The listing builds one solid part. Answer for the finished solid, in the listing's coordinates (mm). Face numbers are marked on the shaded views. Round coordinates to 2 decimals unless told otherwise and drop trailing zeros. Write each loop counter-clockwise with the first axis right and the second up, starting at its lowest first coordinate (ties: lowest second). Pieces come first, ordered by that corner, then holes. Notation, with made-up numbers: M 85.5,-39 L 105.5,-39 A20 ccw 105.5,-33 Z; hole C 16,78.5 d10. An arc over 180 degrees is marked long. One line per item, written item: value. Start each with the question number.
(1) Given P1, Ø8, axis at x = -11.5, z = 9, coming from the -Y side; P2, Ø9.5, axis at x = 22.5, z = 10.5, coming from the -Y side, each flat-ended and moving along its own axis, determine where each tip first touches the part or whether it passes through.
(2) Section A-A (y = -97.5) is taken. Determine the outline of the cut face in (x, z).
(3) Section D-D (z = 29.5) is taken. Determine the outline of the cut face in (x, y).
(4) For a pull along Z with two mould halves and no side action, classify the marked faces 1, 2, 3 and 4 as released by +Z, released by -Z, zero draft, split by the parting line, or undercut.
(5) Section B-B (x = 12) is taken. Determine the outline of the cut face in (y, z).
(6) Consider probe 1 along Y at (x, z) = (-2.5, 4); probe 2 along Y at (x, z) = (12.5, 7); probe 3 along Z at (x, y) = (78.5, -28). Determine where each line is inside the solid, lowest interval first.
(7) Section C-C (y = -52.5) is taken. Determine the outline of the cut face in (x, z), plus the area to 3 significant figures.
```python
from build123d import *

# Parameters (mm, degrees)
F0_W     = 150
F0_H     = 100
F1_DEPTH = 100
F4_DEPTH = 25
F5_SIZE  = 24
F6_R     = 9.380877
F7_DEPTH = 24.5
F8_W     = 13.083855
F8_H     = 15.305644
F9_DEPTH = 25.7


with BuildPart() as f1:
    # F0 (on Front) → F1 (new body)
    with BuildSketch(Plane.XZ):
        with Locations((15.379184, 8.105334)):
            Rectangle(F0_W, F0_H)
    extrude(amount=F1_DEPTH)

    # F3 (on face) → F4 (join)
    with BuildSketch(Plane.XZ.offset(100)):
        with BuildLine():
            ThreePointArc((-14.94097, 58.105334), (10.023203, 33.033909), (35.058928, 58.033884))
            ThreePointArc((35.058928, 58.033884), (35.058903, 58.069609), (35.058826, 58.105334))
            Line((35.058826, 58.105334), (-14.94097, 58.105334))
        make_face()
    extrude(amount=F4_DEPTH)

    # F5
    f5_edges = [f1.edges().sort_by_distance(p)[0] for p in [
        (90.379184, -50, 58.105334),
    ]]
    chamfer(f5_edges, length=F5_SIZE)

    # F6 (on face) → F7 (cut)
    with BuildSketch(Plane.XZ.offset(100)):
        with Locations((19.53912, 7.652821)):
            Circle(F6_R)
    extrude(amount=-F7_DEPTH, mode=Mode.SUBTRACT)

    # F8 (on face) → F9 (cut)
    with BuildSketch(Plane.XZ.offset(100)):
        with Locations((-30.697948, 2.715517)):
            Rectangle(F8_W, F8_H)
    extrude(amount=-F9_DEPTH, mode=Mode.SUBTRACT)


solid = f1.part
```
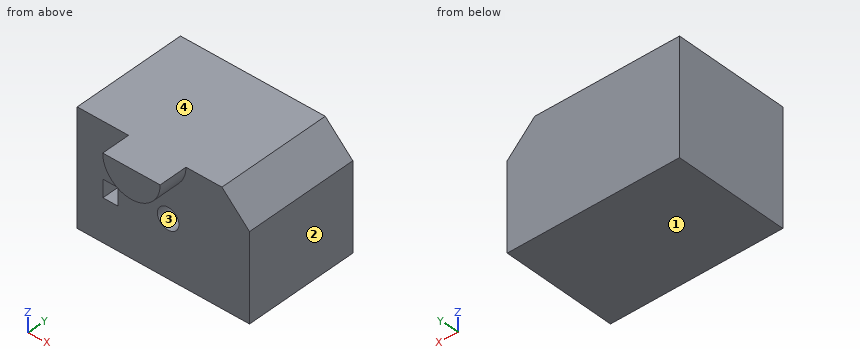
Recorded:
1. P1: stops at y = -100
1. P2: stops at y = -75.5
2. outline: M -59.62,-41.89 L 90.38,-41.89 L 90.38,34.11 L 66.38,58.11 L -59.62,58.11 Z; hole M -37.24,-4.94 L -24.16,-4.94 L -24.16,10.37 L -37.24,10.37 Z; hole C 19.54,7.65 d18.76
3. outline: M -59.62,-100 L 90.38,-100 L 90.38,0 L -59.62,0 Z
4. face 1: released by -Z
4. face 2: zero draft
4. face 3: undercut
4. face 4: released by +Z
5. outline: M -125,33.11 L -100,33.11 L -100,13.24 L -75.5,13.24 L -75.5,2.07 L -100,2.07 L -100,-41.89 L 0,-41.89 L 0,58.11 L -125,58.11 Z
6. probe 1: y = -100 to 0
6. probe 2: y = -75.5 to 0
6. probe 3: z = -41.89 to 45.98
7. outline: M -59.62,-41.89 L 90.38,-41.89 L 90.38,34.11 L 66.38,58.11 L -59.62,58.11 Z
7. area: 14,700 mm2
